Geometry: final body of the model. Coordinates: model frame, mm. Face numbers are marked on the shaded views. A direction names the side the tool comes from. Give positions to 0.01 mm unless a question says otherwise; leave off trailing zeros. Loops run counter-clockwise (first coordinate to the right, second up) from the corner with the lowest first, then second, coordinate; pieces in that order, holes last. Notation, with made-up numbers: (-6.75, 89) - (0.25, 89) arc R28 ccw to (0.25, 125) - close; hole circle Ø9 at (-1, -34.75). An arc over 180 degrees is marked (long way). Use CSV: the item, a comma, the result in double quotes. Start each with the question number.
```python
from build123d import *

# Parameters (mm, degrees)
SKETCH1_W           = 40
SKETCH1_H           = 8.89
SKETCH1_R           = 2.2
BOSS_EXTRUDE1_DEPTH = 6.5
CUT_EXTRUDE1_REACH  = 24.832
SKETCH2_W           = 8
SKETCH2_H           = 3.5
SKETCH2_W_2         = 13
SKETCH3_R           = 5.5
CUT_EXTRUDE2_DEPTH  = 3.5
CUT_EXTRUDE3_DEPTH  = 1.5
SKETCH6_W           = 16
SKETCH6_H           = 3
BOSS_EXTRUDE2_DEPTH = 4


with BuildPart() as part:
    # Sketch1 → Boss-Extrude1 (new body)
    with BuildSketch(Plane(origin=(0, 0, 0), x_dir=(1, 0, 0), z_dir=(0, 1, 0))):
        Rectangle(SKETCH1_W, SKETCH1_H)
        with Locations(Location((0, 0, 0), (0, 0, 90))):
            Circle(SKETCH1_R, mode=Mode.SUBTRACT)
        with Locations(Location((-15, 0, 0), (0, 0, 90))):
            Circle(SKETCH1_R, mode=Mode.SUBTRACT)
        with Locations(Location((15, 0, 0), (0, 0, 90))):
            Circle(SKETCH1_R, mode=Mode.SUBTRACT)
    extrude(amount=BOSS_EXTRUDE1_DEPTH)

    # Cut-Extrude1: up to this face of the body (flat: up to its plane)
    cut_extrude1_end = Plane(part.part.faces().sort_by_distance((0, 3.25, -4.445))[0])
    # Sketch2 → Cut-Extrude1 (cut, up to the picked face)
    with BuildSketch(Plane.XY.offset(4.445), mode=Mode.PRIVATE) as cut_extrude1_sk1:
        with Locations((0, 4.75)):
            Rectangle(SKETCH2_W, SKETCH2_H)
    cut_extrude1_tool1 = split(extrude(cut_extrude1_sk1.sketch, amount=-CUT_EXTRUDE1_REACH, mode=Mode.PRIVATE), bisect_by=cut_extrude1_end, keep=Keep.BOTH, mode=Mode.PRIVATE)
    # Sketch2 → Cut-Extrude1 (cut, up to the picked face)
    with BuildSketch(Plane.XY.offset(4.445), mode=Mode.PRIVATE) as cut_extrude1_sk2:
        with Locations((-13.5, 1.75)):
            Rectangle(SKETCH2_W_2, SKETCH2_H)
    cut_extrude1_tool2 = split(extrude(cut_extrude1_sk2.sketch, amount=-CUT_EXTRUDE1_REACH, mode=Mode.PRIVATE), bisect_by=cut_extrude1_end, keep=Keep.BOTH, mode=Mode.PRIVATE)
    # Sketch2 → Cut-Extrude1 (cut, up to the picked face)
    with BuildSketch(Plane.XY.offset(4.445), mode=Mode.PRIVATE) as cut_extrude1_sk3:
        with Locations((13.5, 1.75)):
            Rectangle(SKETCH2_W_2, SKETCH2_H)
    cut_extrude1_tool3 = split(extrude(cut_extrude1_sk3.sketch, amount=-CUT_EXTRUDE1_REACH, mode=Mode.PRIVATE), bisect_by=cut_extrude1_end, keep=Keep.BOTH, mode=Mode.PRIVATE)
    add(cut_extrude1_tool1.solids().sort_by(Axis((0, 4.75, 4.445), (0, 0, -1)))[0], mode=Mode.SUBTRACT)
    add(cut_extrude1_tool2.solids().sort_by(Axis((-13.5, 1.75, 4.445), (0, 0, -1)))[0], mode=Mode.SUBTRACT)
    add(cut_extrude1_tool3.solids().sort_by(Axis((13.5, 1.75, 4.445), (0, 0, -1)))[0], mode=Mode.SUBTRACT)

    # Sketch3 → Cut-Extrude2 (cut)
    with BuildSketch(Plane(origin=(0, 3, 0), x_dir=(1, 0, 0), z_dir=(0, 1, 0))):
        Circle(SKETCH3_R)
    extrude(amount=CUT_EXTRUDE2_DEPTH, mode=Mode.SUBTRACT)

    # Sketch4 → Cut-Extrude3 (cut)
    with BuildSketch(Plane(origin=(0, 3.5, 0), x_dir=(-1, 0, 0), z_dir=(0, -1, 0))):
        Polygon((12.892671517, 3.65), (10.785343035, 0), (12.892671517, -3.65), (17.107328483, -3.65), (19.214656965, 0), (17.107328483, 3.65), align=None)
        Polygon((-17.107328483, 3.65), (-19.214656965, 0), (-17.107328483, -3.65), (-12.892671517, -3.65), (-10.785343035, 0), (-12.892671517, 3.65), align=None)
    extrude(amount=-CUT_EXTRUDE3_DEPTH, mode=Mode.SUBTRACT)

    # Sketch6 → Boss-Extrude2 (add)
    with BuildSketch(Plane.XY.offset(4.445)):
        with Locations((-12, 5)):
            Rectangle(SKETCH6_W, SKETCH6_H)
        with Locations((12, 5)):
            Rectangle(SKETCH6_W, SKETCH6_H)
    boss_extrude2 = extrude(amount=BOSS_EXTRUDE2_DEPTH)

    # Mirror1: Boss-Extrude2 across plane
    add(boss_extrude2.mirror(Plane.XY))


solid = part.part
```
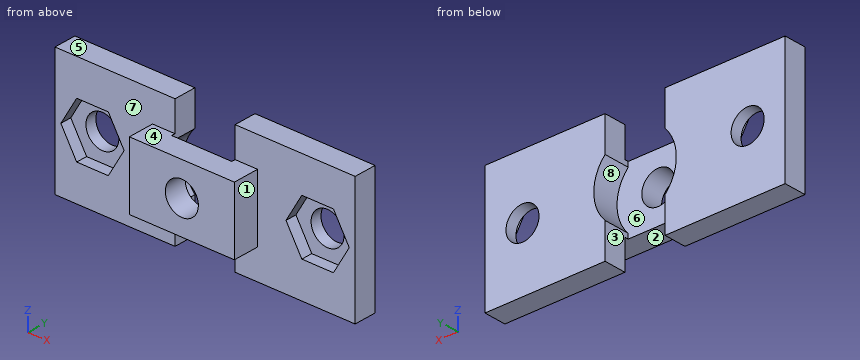
Item 1: Mould query, pull axis Z, two halves, no side actions, for the marked faces 5, 6, 7 and 8. Classes: pulls with the +Z half, pulls with the -Z half, needs draft (parallel to the pull), parting line crosses it, or undercut.
Item 2: Section B-B (z = 6.5). Output: boundary loops of the cut face in (x, y), plus the area to 3 significant figures.
Item 3: Section A-A (x = 0). Output: boundary loops of the cut face in (y, z) (3 decimals).
Item 4: Reachability of the marked faces 1, 2, 3 and 4 from +Z, -Z, +X, -X, +Y, -Y: full face, straight path, thin tool, end or side. Return the list, or none.
Item 5: Pin query (flat end, axial travel): pin 1 Ø1 at (y, z) = (2.5, 0.5) entering from +X; pin 2 Ø5.5 at (x, z) = (0, 0) entering from +Y; pin 3 Ø1.8 at (x, y) = (1, 2) entering from +Z (3 decimals). Return the tip coordinate at first contact, or that it passes through.
Item 6: Ray query, probe 1 along X at (y, z) = (5.4, 0); probe 2 along X at (y, z) = (5, -5.75); probe 3 along Y at (x, z) = (15, 5.25). Return the intervals inside material, ascending.
Item 7: Section C-C (y = 0.75). Output: boundary loops of the cut face in (x, z) (3 decimals).
Item 8: Section D-D (z = 3). Output: boundary loops of the cut face in (x, y), plus the area to 3 significant figures.
Outcome:
1,face 5,"pulls with the +Z half"
1,face 6,"undercut"
1,face 7,"needs draft"
1,face 8,"undercut"
2,outline,"(-20, 3.5) - (-4, 3.5) - (-4, 6.5) - (-20, 6.5) - close; (4, 3.5) - (20, 3.5) - (20, 6.5) - (4, 6.5) - close"
2,area,"96.0 mm2"
3,outline,"(0, -4.445) - (3, -4.445) - (3, -2.2) - (0, -2.2) - close; (0, 2.2) - (3, 2.2) - (3, 4.445) - (0, 4.445) - close"
4,face 1,"+Z, -Z, +X, -Y"
4,face 2,"-Z, +X, -X, -Y"
4,face 3,"+Z, -Z, +Y"
4,face 4,"+Z, +X, -X, -Y"
5,pin 1,"stops at x = 7"
5,pin 2,"stops at y = 3"
5,pin 3,"stops at z = 4.445"
6,probe 1,"x = -20 to -17.2, -12.8 to -5.5, 5.5 to 12.8, 17.2 to 20"
6,probe 2,"x = -20 to -4, 4 to 20"
6,probe 3,"y = 3.5 to 6.5"
7,outline,"(-7, -4.445) - (7, -4.445) - (7, 4.445) - (-7, 4.445) - close; hole circle Ø4.4 at (0, 0)"
8,outline,"(-20, 3.5) - (-17.48, 3.5) - (-17.48, 5) - (-12.52, 5) - (-12.52, 3.5) - (-7, 3.5) - (-7, 0) - (7, 0) - (7, 3.5) - (12.52, 3.5) - (12.52, 5) - (17.48, 5) - (17.48, 3.5) - (20, 3.5) - (20, 6.5) - (4.61, 6.5) - (4.61, 3) - (-4.61, 3) - (-4.61, 6.5) - (-20, 6.5) - close"
8,area,"122 mm2"
